```python
from build123d import *

# Parameters (mm, degrees)
F0_W     = 4.7625
F0_H     = 4.7625
F1_DEPTH = 12.7
F2_R     = 1.27
F3_R     = 3.81
F4_R     = 50.8
F5_R     = 0.635
F6_R     = 2.54
F7_R     = 0.762


with BuildPart() as f1:
    # F0 (on Front) → F1 (new body)
    with BuildSketch(Plane.XZ):
        Polygon((3.175, 9.525), (0, 9.525), (0, 0), (6.35, 0), (6.35, -23.8125), (6.35, -28.575), (6.35, -50.8), (9.525, -50.8), (22.225, -25.4), (82.55, 0), (82.55, 5.450216), (79.375, 5.450216), (79.375, 3.175), (3.175, 3.175), align=None)
        Polygon((9.525, -43.18), (9.525, 0), (16.747011, -25.4), align=None, mode=Mode.SUBTRACT)
        Polygon((14.605, 0), (34.925, 0), (21.733211, -20.196598), align=None, mode=Mode.SUBTRACT)
        Polygon((37.588557, -1.75892), (50.240452, -10.113791), (25.550904, -20.227582), align=None, mode=Mode.SUBTRACT)
        Polygon((40.005, 0), (74.93, 0), (54.61, -8.323855), align=None, mode=Mode.SUBTRACT)
        with Locations((3.96875, -26.19375)):
            Rectangle(F0_W, F0_H)
    extrude(amount=F1_DEPTH)

    # F2
    f2_edges = [f1.edges().sort_by_distance(p)[0] for p in [
        (79.375, -6.35, 3.175),
        (3.175, -6.35, 3.175),
    ]]
    fillet(f2_edges, radius=F2_R)

    # F3
    f3_edges = [f1.edges().sort_by_distance(p)[0] for p in [
        (82.55, -6.35, 0),
        (0, -6.35, 0),
        (9.525, -6.35, -50.8),
    ]]
    fillet(f3_edges, radius=F3_R)

    # F4
    f4_edges = [f1.edges().sort_by_distance(p)[0] for p in [
        (22.225, -6.35, -25.4),
    ]]
    fillet(f4_edges, radius=F4_R)

    # F5
    f5_edges = [f1.edges().sort_by_distance(p)[0] for p in [
        (74.93, -6.35, 0),
        (25.550904, -6.35, -20.227582),
        (50.240452, -6.35, -10.113791),
        (9.525, -6.35, 0),
        (9.525, -6.35, -43.18),
        (14.605, -6.35, 0),
        (34.925, -6.35, 0),
        (40.005, -6.35, 0),
        (21.733211, -6.35, -20.196598),
    ]]
    fillet(f5_edges, radius=F5_R)

    # F6
    f6_edges = [f1.edges().sort_by_distance(p)[0] for p in [
        (16.747011, -6.35, -25.4),
        (37.588557, -6.35, -1.75892),
        (54.61, -6.35, -8.323855),
    ]]
    fillet(f6_edges, radius=F6_R)

    # F7
    f7_edges = [f1.edges().sort_by_distance(p)[0] for p in [
        (0, -6.35, 9.525),
        (3.175, -6.35, 9.525),
        (1.5875, -6.35, -23.8125),
        (1.5875, -6.35, -28.575),
        (1.5875, -12.7, -26.19375),
        (1.5875, 0, -26.19375),
    ]]
    fillet(f7_edges, radius=F7_R)


solid = f1.part
```
Can you work these out from the model? Positions are in its coordinate system, mm. A direction names the side the tool comes from. Give positions to 0.01 mm unless a question says otherwise; leave off trailing zeros. Write each loop counter-clockwise with the first axis right and the second up, starting at its lowest first coordinate (ties: lowest second). Pieces come first, ordered by that corner, then holes. Notation, with made-up numbers: (29, 74) - (83, 74) arc R25 ccw to (83, 88) - close; hole circle Ø9 at (-9.75, 44). An arc over 180 degrees is marked (long way). Write item = value, one per line. Start each with the question number.
1. Imagine slicing it at C-C (x = 25.5). Please give me the cut outline in (y, z) (3 decimals).
2. Imagine slicing it at A-A (z = -38). Please give me the cut outline in (x, y) (3 decimals), and give its area (3 significant figures).
3. For pin 1 (1 mm diameter, centred on x = 80.5, y = -6.5, fed in from +Z); pin 2 (4 mm diameter, centred on x = 10.5, y = -10, fed in from +Z) (3 decimals); pin 3 (4 mm diameter, centred on x = 55.5, y = -5.5, fed in from -Z), each with a flat end and sliding along its axis, tell me the tip position at first contact or that it passes through.
4. Imagine slicing it at B-B (z = -14.5). Count the separate pieces of the cut face and the enclosed holes in it, and give its area (3 significant figures).
5. Thinking about a two-plate mould opening in X: for faces 1 (the face through (57, -6, 0)), 2 (the face through (24.71, -6.439, -27.683)), 3 (the face through (0, -6, 6)), which applies, released by +X, released by -X, zero draft, split by the parting line, or undercut?
6. Imagine slicing it at D-D (z = -6). Please give me the cut outline in (x, y) (3 decimals), and give its area (3 significant figures).
7. Please list where these lines run through material, in increasing order: line 1 (Z direction, x = 45.5, y = -10.5) (3 decimals); line 2 (X direction, y = -10.25, z = -19) (3 decimals); line 3 (X direction, y = -8.5, z = -2).
8. On a 3-axis mill with a long thin cutter (end or side, diameter ignored), from which of +Z, -Z, +X, -X, +Y, -Y can I reach the whole of each face in a straight line? I mean faces 4 (the face through (6.35, -6, -12)), 5 (the face through (1.588, -6, -26)), 6 (the face through (42, -6, 3.175)), 7 (the face through (16.6, -6.4, -25.4)). Say none if no direction works.
Worked answers:
q1.outline = (-12.7, -26.965) - (0, -26.965) - (0, -14.43) - (-12.7, -14.43) - close; (-12.7, 0) - (0, 0) - (0, 3.175) - (-12.7, 3.175) - close
q2.outline = (6.35, -12.7) - (9.525, -12.7) - (9.525, 0) - (6.35, 0) - close; (11.629, -12.7) - (16.181, -12.7) - (16.181, 0) - (11.629, 0) - close
q2.area = 98.1 mm2
q3.pin_1 = 5.45
q3.pin_2 = 3.175
q3.pin_3 = -12.23
q4.separate_pieces = 4
q4.enclosed_holes = 0
q4.area = 275 mm2
q5.face_1 = undercut
q5.face_2 = released by +X
q5.face_3 = released by -X
q6.outline = (6.35, -12.7) - (9.525, -12.7) - (9.525, 0) - (6.35, 0) - close; (11.231, -12.7) - (16.723, -12.7) - (16.723, 0) - (11.231, 0) - close; (31.006, -12.7) - (34.824, -12.7) - (34.824, 0) - (31.006, 0) - close; (44.011, -12.7) - (50.533, -12.7) - (50.533, 0) - (44.011, 0) - close; (60.283, -12.7) - (68.3, -12.7) - (68.3, 0) - (60.283, 0) - close
q6.area = 343 mm2
q7.line_1 = -15.6 to -12.056, -6.983 to -3.132, 0 to 3.175
q7.line_2 = 6.35 to 9.525, 14.927 to 21.311, 22.515 to 26.574, 28.548 to 37.546
q7.line_3 = 6.35 to 15.31, 33.62 to 43.51, 70.05 to 77.8
q8.face_4 = -X, +Y, -Y
q8.face_5 = -Z, -X, +Y, -Y
q8.face_6 = +Z, +Y, -Y
q8.face_7 = +Y, -Y
